Geometry check sheet. Reference: the model listing, model coordinates, mm. Give positions to 0.01 mm unless a question says otherwise; leave off trailing zeros. Order: outer loops, then holes, each group sorted by start corner. A loop starts at its lowest first (then second) coordinate and runs counter-clockwise, first axis right, second up.
Autodesk Inventor part; units mm, degrees
ref_plane "YZ Plane" through (0, 0, 0) normal (1, 0, 0) x (0, 1, 0)
ref_plane "XZ Plane" through (0, 0, 0) normal (0, 1, 0) x (-1, 0, 0)
ref_plane "XY Plane" through (0, 0, 0) normal (0, 0, 1) x (1, 0, 0)
sketch "Boceto1" plane through (0, 0, 0) normal (1, 0, 0) x (0, 1, 0)
  circle A0 centre (0, 0) radius 2
  arc A1 (5, 0) -> (-5, 0) centre (0, 0) ccw
  circle A2 centre (0, -140) radius 3.175
  arc A3 (-7.4952, -139.7322) -> (7.4952, -139.7322) centre (0, -140) ccw
  line L0 (5, 0) -> (7.5, -140)
  line L1 (-5, 0) -> (-7.5, -140)
  dimension "d0" = 4
  dimension "d1" = 10
  dimension "d2" = 6.35
  dimension "d3" = 140
  dimension "d4" = 15
extrude "Extrusión1" add sketch "Boceto1" along normal blind 3
properties part number "Transmision_Sup"
Q1. Cross-section at C-C, the plane z = -100.5. Record the boundary of the cut face in (x, y), and give its area (3 significant figures).
Q2. Gauge pin test, flat end, axial feed: P1, Ø1.5, axis at x = 2, y = 1, coming from the -Z side. Record the tip position at first contact, or that the pin passes through.
Q3. Thickness scan on L1, parallel to Y at x = 1.6, z = -140 (3 decimals); L2, parallel to Z at x = 2.3, y = -1.5; L3, parallel to Y at x = 2.3, z = -125. Record the ranges inside material, lowest first.
Q4. Cross-section at D-D, the plane z = -46. Record the boundary of the cut face in (x, y), and give its area (3 significant figures).
Q5. Cross-section at B-B, the plane x = 0.5. Record the boundary of the cut face in (y, z) (3 decimals).
Q6. Cross-section at A-A, the plane y = 0. Record the boundary of the cut face in (x, z) (3 decimals).
Q7. Release check for a two-part mould opening along Z. For faces 1 (the face through (0, 0, -70)), 2 (the face through (1, 0, 2)), 3 (the face through (1, 0, 5)) record: pulls with the +Z half, pulls with the -Z half, needs draft (parallel to the pull), parting line crosses it, or undercut.
Answers follow:
1. outline: (0, -6.79) - (3, -6.79) - (3, 6.79) - (0, 6.79) - close
1. area: 40.8 mm2
2. P1: stops at z = -147.5
3. L1: y = -7.5 to -3.175, 3.175 to 7.5
3. L2: z = -147.35 to -142.8, -137.2 to -1.32, 1.32 to 4.77
3. L3: y = -7.23 to 7.23
4. outline: (0, -5.82) - (3, -5.82) - (3, 5.82) - (0, 5.82) - close
4. area: 34.9 mm2
5. outline: (-7.495, -139.732) arc R7.5 ccw (long way) to (7.495, -139.732) - (5, 0) arc R5 ccw to (-5, 0) - close; hole circle Ø6.35 at (0, -140); hole circle Ø4 at (0, 0)
6. outline: (0, -147.5) - (3, -147.5) - (3, -143.175) - (0, -143.175) - close; (0, -136.825) - (3, -136.825) - (3, -2) - (0, -2) - close; (0, 2) - (3, 2) - (3, 5) - (0, 5) - close
7. face 1: needs draft
7. face 2: undercut
7. face 3: pulls with the +Z half
